Input: part model. Units: mm. Frame: model coordinates. A direction names the side the tool comes from. Coordinates: 2 decimals unless noted, no trailing zeros. Write each loop counter-clockwise with the first axis right and the second up, starting at its lowest first coordinate (ties: lowest second). Pieces come first, ordered by that corner, then holes. Notation, with made-up numbers: M -6.75,33 L 42.25,33 A27 cw 42.25,66 Z; hole C 44.5,-30.75 d11. An arc over 180 degrees is marked long. Use one line per item in the form item = value.
Autodesk Inventor part; units mm, degrees
ref_plane "YZ Plane" through (0, 0, 0) normal (1, 0, 0) x (0, 1, 0)
ref_plane "XZ Plane" through (0, 0, 0) normal (0, 1, 0) x (-1, 0, 0)
ref_plane "XY Plane" through (0, 0, 0) normal (0, 0, 1) x (1, 0, 0)
sketch "草图1" plane through (0, 0, 0) normal (0, 1, 0) x (-1, 0, 0)
  circle A0 centre (0, 0) radius 1.5
  line L0 (0, 0) -> (-50, 0) construction
  circle A1 centre (-50, 0) radius 1.5
  line L1 (5, -5) -> (-55, -5)
  line L2 (-55, -5) -> (-55, 5)
  line L3 (-55, 5) -> (5, 5)
  line L4 (5, 5) -> (5, -5)
  line L5 (-25, 0) -> (-25, -6.3237) construction
  dimension "d0" = 3
  dimension "d1" = 50
  dimension "d2" = 3
  dimension "d3" = 10
  dimension "d4" = 60
extrude "拉伸1" add sketch "草图1" along normal blind 6
sketch "草图2" plane through (0, 6, 0) normal (0, 1, 0) x (1, 0, 0)
  line L0 (-5, -5) -> (55, -5)
  line L1 (55, -5) -> (55, 5)
  line L2 (55, 5) -> (-5, 5)
  line L3 (-5, 5) -> (-5, -5)
  circle A0 centre (50, 0) radius 1.5
  circle A1 centre (0, 0) radius 1.5
  line L4 (55, 5) -> (-5, 5)
  line L5 (-5, -5) -> (55, -5)
  line L6 (17, 5) -> (22, 5)
  line L7 (22, 5) -> (22, -5)
  line L8 (22, -5) -> (17, -5)
  line L9 (17, -5) -> (17, 5)
  line L10 (28, 5) -> (33, 5)
  line L11 (33, 5) -> (33, -5)
  line L12 (33, -5) -> (28, -5)
  line L13 (28, -5) -> (28, 5)
  line L14 (25, -5) -> (25, 2.8466) construction
  line L15 (17, -5) -> (22, -5)
  line L16 (22, -5) -> (22, -29.5)
  line L17 (22, -29.5) -> (17, -29.5)
  line L18 (17, -29.5) -> (17, -5)
  line L19 (33, -5) -> (28, -5)
  line L20 (28, -5) -> (28, -29.5)
  line L21 (28, -29.5) -> (33, -29.5)
  line L22 (33, -29.5) -> (33, -5)
  point P0 (28, 5)
  point P1 (28, -5)
  point P2 (33, -5)
  point P3 (33, 5)
  point P4 (17, 5)
  point P5 (22, 5)
  point P6 (33, -5)
  dimension "d7" = 5
  dimension "d8" = 6
  dimension "d24" = 24.5
extrude "拉伸2" add sketch "草图2" along normal blind 10 contours L9 L2 L7 L0 | L0 L16 L17 L18 | L7 L2 L13 L0 | L13 L2 L11 L0 | L0 L22 L21 L20
chamfer "倒角1" distance 2 angle 45 2 edges at (1.5, 6, 0) (51.5, 6, 0)
sketch "草图4" plane through (33, 6, 29.5) normal (1, 0, 0) x (0, 0, -1)
  circle A0 centre (5, 5) radius 2
  line L0 (0, 0) -> (0, 10)
  line L1 (0, 5) -> (5, 5)
  point P0 (29.5, -6)
  dimension "d25" = 4
  dimension "d26" = 5
extrude "拉伸4" cut sketch "草图4" against normal through all
fillet "圆角7" radius 5 4 edges at (30.5, 16, 29.5) (19.5, 16, 29.5) (19.5, 6, 29.5) (30.5, 6, 29.5)
sketch "草图5" plane through (0, 6, 0) normal (0, -1, 0) x (1, 0, 0)
  line L0 (17, 24.5) -> (22, 24.5)
  line L1 (17, 5) -> (17, 24.5)
  line L2 (17, 5) -> (22, 5)
  line L3 (22, 24.5) -> (22, 5)
  line L4 (28, 24.5) -> (33, 24.5)
  line L5 (28, 5) -> (28, 24.5)
  line L6 (28, 5) -> (33, 5)
  line L7 (33, 24.5) -> (33, 5)
  line L8 (17, 19.5) -> (33, 19.5)
  line L9 (33, 24.5) -> (33, 5)
  line L10 (-5, 5) -> (55, 5)
  point P0 (0, 0)
  point P1 (22, 19.5)
  point P2 (28, 19.5)
  dimension "d30" = 14.5
extrude "拉伸5" add sketch "草图5" along normal blind 6 contours L8 L3 L2 L1 | L8 L7 L6 L5
sketch "草图6" plane through (0, 0, 0) normal (0, -1, 0) x (1, 0, 0)
  line L0 (-5, 5) -> (17, 5)
  line L1 (-5, -5) -> (-5, 5)
  line L2 (55, -5) -> (-5, -5)
  line L3 (55, 5) -> (55, -5)
  line L4 (33, 5) -> (55, 5)
  line L5 (33, 5) -> (33, 19.5)
  line L6 (33, 19.5) -> (28, 19.5)
  line L7 (28, 19.5) -> (28, 5)
  line L8 (22, 5) -> (28, 5)
  line L9 (22, 5) -> (22, 19.5)
  line L10 (22, 19.5) -> (17, 19.5)
  line L11 (17, 19.5) -> (17, 5)
  circle A0 centre (50, 0) radius 1.5
  circle A1 centre (0, 0) radius 1.5
  line L12 (17, 19.5) -> (17, 5)
  line L13 (17, 15) -> (33, 15)
  line L14 (33, 5) -> (33, 19.5)
  line L15 (17, 5) -> (33, 5)
  point P0 (28, 15)
  point P1 (22, 15)
  dimension "d34" = 10
extrude "拉伸6" add sketch "草图6" along normal blind 3 contours L11 L13 L9 L15 | L7 L13 L5 L15
ref_plane "工作平面1" through (33, 11, 24.5) normal (1, 0, 0) x (0, 0, -1)
sketch "草图7" plane through (33, 11, 24.5) normal (1, 0, 0) x (0, 0, -1)
  circle A0 centre (0, 0) radius 2
  line L0 (8.5, 1.5) -> (16.5, 1.5)
  line L1 (16.5, 1.5) -> (16.5, -7.5)
  line L2 (16.5, -7.5) -> (8.5, -7.5)
  line L3 (8.5, -7.5) -> (8.5, 1.5)
  point P0 (24.5, -11)
  dimension "d43" = 8
  dimension "d44" = 9
extrude "拉伸7" cut sketch "草图7" against normal through all contours L0 L1 L2 L3
sketch "草图8" plane through (55, 0, -5) normal (0, 0, -1) x (-1, 0, 0)
  line L0 (0, 0) -> (60, 0)
  line L1 (60, 0) -> (60, 6)
  line L2 (38, 6) -> (60, 6)
  line L3 (38, 6) -> (38, 16)
  line L4 (22, 16) -> (38, 16)
  line L5 (22, 6) -> (22, 16)
  line L6 (0, 6) -> (22, 6)
  line L7 (0, 0) -> (0, 6)
  line L8 (22, 6) -> (22, 16)
  line L9 (38, 0) -> (38, -3)
  line L10 (22, 16) -> (38, 16)
  line L11 (38, 16) -> (38, 0)
  line L12 (38, 0) -> (22, 0)
  line L13 (22, 0) -> (22, 16)
  circle A0 centre (30, 8) radius 4
  line L14 (30, 8) -> (30, 0) construction
  line L15 (30, 8) -> (22, 8) construction
  line L16 (0, 0) -> (60, 0)
  point P0 (55, 0)
  dimension "d50" = 8
extrude "拉伸8" cut sketch "草图8" against normal through all contours L7 L6 L13 L0 | L11 L2 L1 L0 | A0
properties part number "合页01"
(1) Pull-direction query (Z, two-part tool) for faces 4 (the flat face through (33, 8, 4)), 5 (the flat face through (20, 3.5, 12)), 6 (the cylindrical face through (19.46, 14.5, 28.07)); classes: pulls with the +Z half, pulls with the -Z half, needs draft (parallel to the pull), parting line crosses it, or undercut.
Computed:
face_4 = needs draft
face_5 = undercut
face_6 = pulls with the +Z half
(2) Section query B-B on z = 5.5. Return the cut outline in (x, y), plus the area to 3 significant figures.
Computed:
outline = M 17,-3 L 22,-3 L 22,5.35 A4 cw 22,10.65 L 22,16 L 17,16 Z; M 28,-3 L 33,-3 L 33,16 L 28,16 L 28,10.65 A4 cw 28,5.35 Z
area = 183 mm^2
(3) First-contact query: pin 1 Ø2.5 at (x, y) = (29.5, -2) entering from +Z; pin 2 Ø5.5 at (x, y) = (19.5, 2.5) entering from +Z; pin 3 Ø4.5 at (x, y) = (24.5, 3) entering from +Z. Flat tips, straight axial feed; report the tip coordinate or a pass-through.
Computed:
pin_1 = 15
pin_2 = 19.5
pin_3 = 5
(4) Section query D-D on x = 20. State how many separate pieces and enclosed holes the cut face has, plus the area to 3 significant figures.
Computed:
separate_pieces = 1
enclosed_holes = 2
area = 427 mm^2
(5) Set-up query: faces 1 (the flat face through (30, 3, 19.5)), 2 (the cylindrical face through (29, 8, 21)), 3 (the flat face through (22, 1, 12)). Return all of +Z, -Z, +X, -X, +Y, -Y with unobstructed straight access to the full face (end or side cutting, diameter ignored); none if empty.
Computed:
face_1 = +Z, +X, -X, -Y
face_2 = +Z, -Z
face_3 = +Z, +Y, -Y
(6) Line query: probe 1 along Z at (x, y) = (31.5, 11); probe 2 along Y at (x, z) = (25, -0.25); probe 3 along X at (y, z) = (2, 19). Output: solid intervals per line, ascending.
Computed:
probe_1 = -5 to 8, 16 to 22.5, 26.5 to 29.5
probe_2 = 0 to 4, 12 to 16
probe_3 = 17 to 22, 28 to 33
(7) Section query A-A on x = 25. Return the cut outline in (y, z).
Computed:
outline = M 0,-5 L 4,-5 L 4,5 L 0,5 Z; M 12,-5 L 16,-5 L 16,5 L 12,5 Z
(8) Section query C-C on y = -2. Return the cut outline in (x, z).
Computed:
outline = M 17,5 L 22,5 L 22,15 L 17,15 Z; M 28,5 L 33,5 L 33,15 L 28,15 Z
